Source: CAD feature listing. Evaluate the final solid. Frame: model axes, mm. Face numbers are marked on the shaded views. A direction names the side the tool comes from. Give positions to 0.01 mm unless a question says otherwise; leave off trailing zeros. Write each loop counter-clockwise with the first axis right and the second up, starting at its lowest first coordinate (ties: lowest second). Pieces come first, ordered by that corner, then holes.
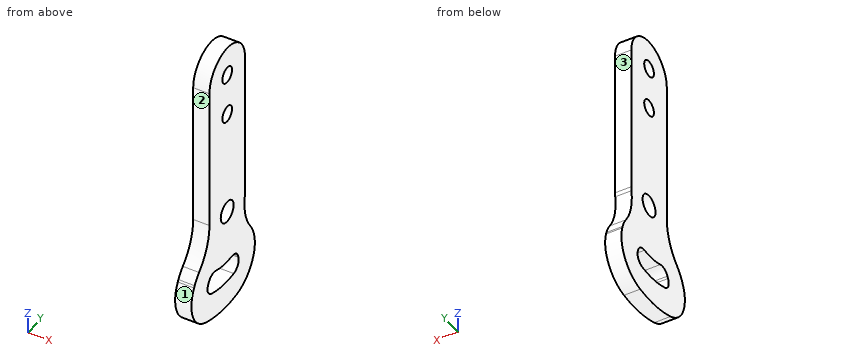
```python
from build123d import *

# Parameters (mm, degrees)
SKETCH1_R           = 1.5
SKETCH1_R_2         = 2
BOSS_EXTRUDE1_DEPTH = 3
FILLET1_R           = 10


with BuildPart() as part:
    # Sketch1 → Boss-Extrude1 (new body)
    with BuildSketch(Plane(origin=(0, 0, 0), x_dir=(0, 0, -1), z_dir=(1, 0, 0))):
        with BuildLine():
            Line((0, 5.5), (28, 5.5))
            ThreePointArc((28, 5.5), (33.5, 0), (28, -5.5))
            Line((28, -5.5), (0, -5.5))
            ThreePointArc((0, -5.5), (-5.5, 0), (0, 5.5))
        make_face()
        Circle(SKETCH1_R, mode=Mode.SUBTRACT)
        with Locations((8, 0)):
            Circle(SKETCH1_R, mode=Mode.SUBTRACT)
        with Locations((28, 0)):
            Circle(SKETCH1_R_2, mode=Mode.SUBTRACT)
        with BuildLine():
            Line((38.004070302, 8.178085192), (38.391808013, 8.292938334))
            ThreePointArc((38.391808013, 8.292938334), (43.99239408, 7.498029345), (47.053808263, 2.741330092))
            ThreePointArc((47.053808263, 2.741330092), (47.144546486, -2.012172918), (46.067482263, -6.642934944))
            ThreePointArc((46.067482263, -6.642934944), (42.08399394, -10.659185108), (36.440523244, -10.272296109))
            Line((36.440523244, -10.272296109), (36.085137843, -10.07933758))
            ThreePointArc((36.085137843, -10.07933758), (32.972810208, -6.517601461), (32.936227504, -1.787780197))
            ThreePointArc((32.936227504, -1.787780197), (33.221239951, -0.548774432), (33.200059493, 0.722413504))
            ThreePointArc((33.200059493, 0.722413504), (34.219227914, 5.341270853), (38.004070302, 8.178085192))
        make_face()
        with BuildLine():
            Line((39.424147025, 3.383986517), (39.811884737, 3.49883966))
            ThreePointArc((39.811884737, 3.49883966), (41.294392813, 3.288422575), (42.104767156, 2.029296302))
            ThreePointArc((42.104767156, 2.029296302), (42.171937009, -1.489530602), (41.374629727, -4.917497297))
            ThreePointArc((41.374629727, -4.917497297), (40.320176936, -5.98062234), (38.826317046, -5.878210546))
            Line((38.826317046, -5.878210546), (38.470931645, -5.685252017))
            ThreePointArc((38.470931645, -5.685252017), (37.647080212, -4.742439515), (37.637396555, -3.490428004))
            ThreePointArc((37.637396555, -3.490428004), (38.193849428, -1.071416748), (38.152497105, 1.410426365))
            ThreePointArc((38.152497105, 1.410426365), (38.422276981, 2.633065075), (39.424147025, 3.383986517))
        make_face(mode=Mode.SUBTRACT)
    extrude(amount=BOSS_EXTRUDE1_DEPTH)

    # Fillet1
    fillet1_edges = [part.edges().sort_by_distance(p)[0] for p in [
        (1.5, -2.978897206, -32.623437188),
        (1.5, 1.952534512, -33.141751548),
    ]]
    fillet(fillet1_edges, radius=FILLET1_R)


solid = part.part
```
1. Contact query for flat-ended pins moving along their axis: P1, Ø3.5, axis at y = 0, z = -28, coming from the -X side; P2, Ø1, axis at x = 2, z = -6.5, coming from the +Y side; P3, Ø1.5, axis at x = 2, z = -14.5, coming from the -Y side. Output: stop coordinate, or through.
2. Cut plane A-A, the plane y = 0. Return the cut outline in (x, z), then the cut area to 3 significant figures.
3. Cut plane D-D, the plane z = -24. Return the cut outline in (x, y), then the cut area to 3 significant figures.
4. Cut plane B-B, the plane z = -8. Return the cut outline in (x, y).
5. Cut plane C-C, the plane x = 0.6. State how many separate pieces and enclosed holes the cut face has, then the cut area to 3 significant figures.
6. Line query: L1, parallel to Y at x = 2.15, z = 0; L2, parallel to Y at x = 0.8, z = -10; L3, parallel to Z at x = 0.5, y = 0.25. Output: solid intervals per line, ascending.
7. Access query for the marked faces 1, 2 and 3. Directions: +Z, -Z, +X, -X, +Y, -Y. A direction counts if a zero-diameter tool reaches every point of the face in a straight line with its end or side. Return the directions, or none.
Response values:
1. P1: passes through
1. P2: stops at y = 5.5
1. P3: stops at y = -5.5
2. outline: (0, -47.25) - (3, -47.25) - (3, -42.25) - (0, -42.25) - close; (0, -38.25) - (3, -38.25) - (3, -30) - (0, -30) - close; (0, -26) - (3, -26) - (3, -9.5) - (0, -9.5) - close; (0, -6.5) - (3, -6.5) - (3, -1.5) - (0, -1.5) - close; (0, 1.5) - (3, 1.5) - (3, 5.5) - (0, 5.5) - close
2. area: 116 mm2
3. outline: (0, -5.5) - (3, -5.5) - (3, 5.5) - (0, 5.5) - close
3. area: 33.0 mm2
4. outline: (0, -5.5) - (3, -5.5) - (3, -1.5) - (0, -1.5) - close; (0, 1.5) - (3, 1.5) - (3, 5.5) - (0, 5.5) - close
5. separate pieces: 1
5. enclosed holes: 4
5. area: 589 mm2
6. L1: y = -5.5 to -1.5, 1.5 to 5.5
6. L2: y = -5.5 to 5.5
6. L3: z = -47.25 to -42.25, -38.25 to -29.98, -26.02 to -9.48, -6.52 to -1.48, 1.48 to 5.49
7. face 1: +X, -X, -Y
7. face 2: +Z, +X, -X, -Y
7. face 3: +Z, +X, -X, +Y
